from build123d import *

# Parameters (mm, degrees)
SKETCH1_R           = 2
SKETCH1_W           = 20.5
SKETCH1_H           = 40.5
BOSS_EXTRUDE1_DEPTH = 3


with BuildPart() as part:
    # Sketch1 → Boss-Extrude1 (new body)
    with BuildSketch(Plane(origin=(0, 0, 0), x_dir=(1, 0, 0), z_dir=(0, 1, 0))):
        Polygon((-45, 10), (-45, 2.5), (-50, 2.5), (-50, -7.5), (-45, -7.5), (-45, -15), (-50, -15), (-50, -25), (-45, -25), (-45, -32.5), (-50, -32.5), (-50, -40), (50, -40), (50, -32.5), (45, -32.5), (45, -25), (50, -25), (50, -15), (45, -15), (45, -7.5), (50, -7.5), (50, 2.5), (45, 2.5), (45, 10), (50, 10), (50, 15), (45, 15), (19, 35), (-19, 35), (-45, 15), (-50, 15), (-50, 10), align=None)
        with Locations(Location((0, 30, 0), (0, 0, 270))):
            Circle(SKETCH1_R, mode=Mode.SUBTRACT)
        with Locations(Location((-36, -12, 0), (0, 0, 270))):
            Circle(SKETCH1_R, mode=Mode.SUBTRACT)
        with Locations(Location((36, -12, 0), (0, 0, 270))):
            Circle(SKETCH1_R, mode=Mode.SUBTRACT)
        with Locations((-15.05, -9.75)):
            Rectangle(SKETCH1_W, SKETCH1_H, mode=Mode.SUBTRACT)
    extrude(amount=BOSS_EXTRUDE1_DEPTH)


solid = part.part
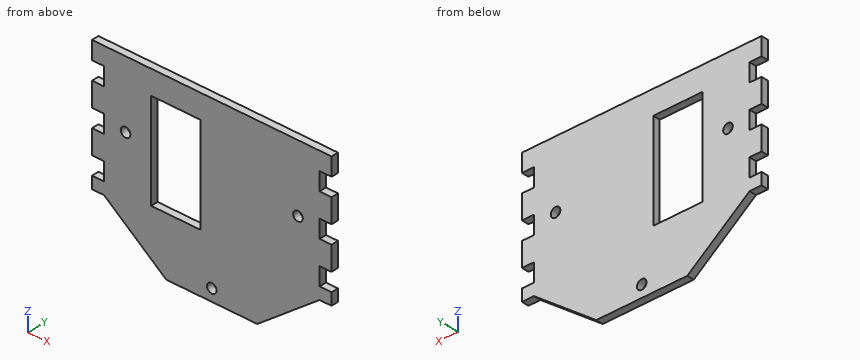
Check sheet for the modelled part. Datum: model origin and axes. Units: mm. Round coordinates to 2 decimals unless told otherwise and drop trailing zeros. Loops run counter-clockwise (first coordinate to the right, second up) from the corner with the lowest first, then second, coordinate; pieces in that order, holes last. Notation, with made-up numbers: (42.25, -25.5) -> (65.25, -25.5) arc R17 cw to (65.25, -16.5) -> close; hole circle Ø3 at (7, 65.5). An arc over 180 degrees is marked (long way). Put each result on its own line as item: value. Start each with the question number.
1. Section check C-C (y = 0.5). Give the number of separate pieces and of enclosed holes in the cut face, plus the area to 3 significant figures.
2. Gauge pin test, flat ends, axial feed: pin 1 (0.9 mm diameter, centred on x = 48.5, y = 1.5, fed in from -Z); pin 2 (1.5 mm diameter, centred on y = 2.5, z = -23.5, fed in from -X) (3 decimals); pin 3 (1.5 mm diameter, centred on y = 2, z = 9.5, fed in from -X); pin 4 (2.5 mm diameter, centred on x = 0, z = -30, fed in from +Y). Record the tip position at first contact, or that the pin passes through.
3. Section check B-B (x = -8). Enter the section's corners in (y, z).
4. Section check D-D (x = 43.5). Enter the section's corners in (y, z).
5. Scan lines: probe 1 along X at (y, z) = (1.6, 12); probe 2 along X at (y, z) = (2.05, 28); probe 3 along Z at (x, y) = (-13, 1.15). Record each from-to range of solid material in increasing order.
6. Section check A-A (z = 17.5). Enter the section's corners in (x, y), plus the area to 4 significant figures.
Findings:
1. separate pieces: 1
1. enclosed holes: 4
1. area: 5,690 mm^2
2. pin 1: stops at z = -15
2. pin 2: stops at x = -34.925
2. pin 3: stops at x = -45
2. pin 4: passes through
3. outline: (0, -35) -> (3, -35) -> (3, -10.5) -> (0, -10.5) -> close; (0, 30) -> (3, 30) -> (3, 40) -> (0, 40) -> close
4. outline: (0, -16.15) -> (3, -16.15) -> (3, 40) -> (0, 40) -> close
5. probe 1: x = -45 to -38, -34 to -25.3, -4.8 to 34, 38 to 45
5. probe 2: x = -45 to -25.3, -4.8 to 45
5. probe 3: z = -35 to -10.5, 30 to 40
6. outline: (-50, 0) -> (-25.3, 0) -> (-25.3, 3) -> (-50, 3) -> close; (-4.8, 0) -> (50, 0) -> (50, 3) -> (-4.8, 3) -> close
6. area: 238.5 mm^2
